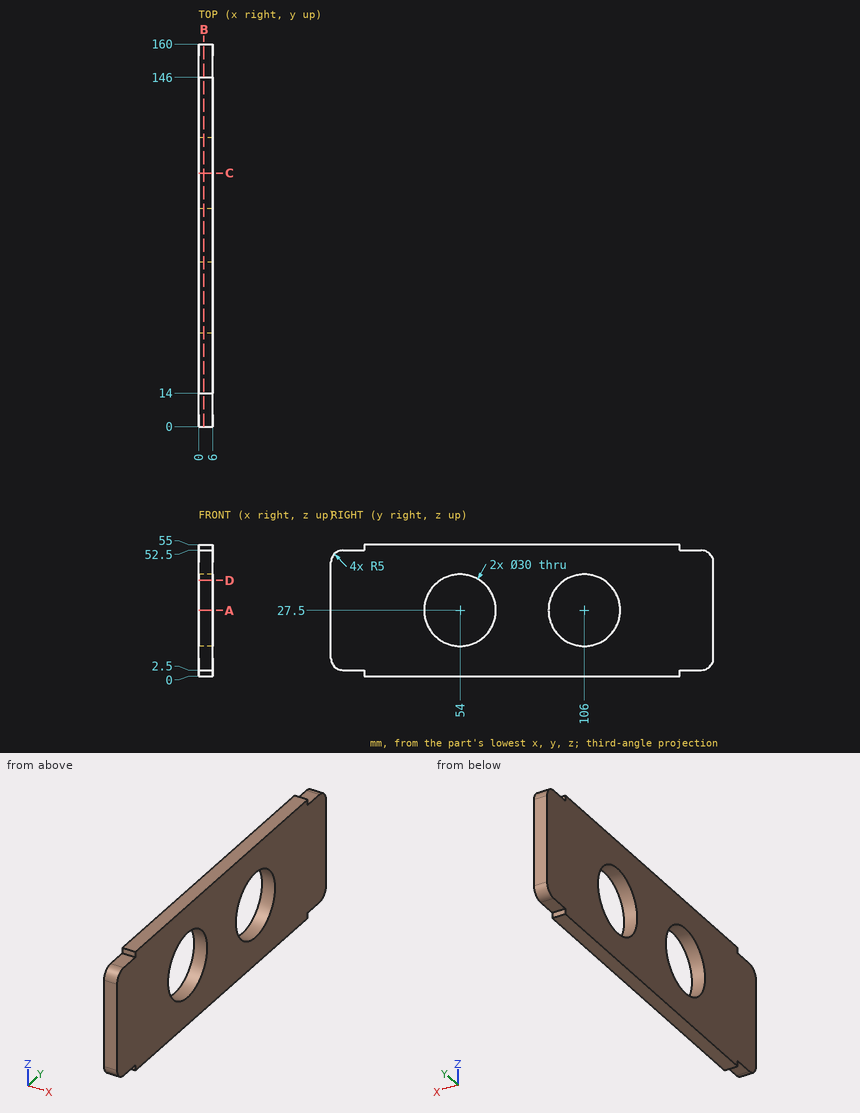
Part print with two shaded views. Sizes in mm from the minimum x, y, z corner. Coordinates: 2 decimals unless noted, no trailing zeros. Write each loop counter-clockwise with the first axis right and the second up, starting at its lowest first coordinate (ties: lowest second). Pieces come first, ordered by that corner, then holes. Notation, with made-up numbers: (55, 79.25) -> (81, 79.25) arc R24 cw to (81, 93.25) -> close; hole circle Ø9 at (84, -4). An arc over 180 degrees is marked (long way). Return JSON: item names as keys, results as strings. Group by question number.
Q1. Cut at B-B, the plane x = 2.2. Give the cut face in (y, z), then the cut area to 3 significant figures.
Q2. Cut at A-A, the plane z = 27.5. Give the cut face in (x, y).
Q3. Cut at D-D, the plane z = 40. Give the cut face in (x, y).
Q4. Drill centre lines: line 1 (Y direction, x = 2.3, z = 28); line 2 (Y direction, x = 4.25, z = 22.5); line 3 (Z direction, x = 3.95, y = 105). Where is each one in solid material? Low to high.
Q5. Cut at C-C, the plane y = 106. Give the cut face in (x, z), then the cut area to 3 significant figures.
Q6. Flat gauge pins, fed straight in: pin 1 (3 mm diameter, centred on x = 2.5, y = 150.5, fed in from -Z); pin 2 (18 mm diameter, centred on y = 106, z = 27.5, fed in from +X); pin 3 (0.8 mm diameter, centred on x = 3, z = 54, fed in from +Y); pin 4 (1.2 mm diameter, centred on x = 3, z = 54, fed in from -Y). Where does each tip first touch, or does it go through?
Returned:
{
 "1": {"outline": "(0, 7.5) arc R5 ccw to (5, 2.5) -> (14, 2.5) -> (14, 0) -> (146, 0) -> (146, 2.5) -> (155, 2.5) arc R5 ccw to (160, 7.5) -> (160, 47.5) arc R5 ccw to (155, 52.5) -> (146, 52.5) -> (146, 55) -> (14, 55) -> (14, 52.5) -> (5, 52.5) arc R5 ccw to (0, 47.5) -> close; hole circle Ø30 at (54, 27.5); hole circle Ø30 at (106, 27.5)", "area": "7,220 mm2"},
 "2": {"outline": "(0, 0) -> (6, 0) -> (6, 39) -> (0, 39) -> close; (0, 69) -> (6, 69) -> (6, 91) -> (0, 91) -> close; (0, 121) -> (6, 121) -> (6, 160) -> (0, 160) -> close"},
 "3": {"outline": "(0, 0) -> (6, 0) -> (6, 45.71) -> (0, 45.71) -> close; (0, 62.29) -> (6, 62.29) -> (6, 97.71) -> (0, 97.71) -> close; (0, 114.29) -> (6, 114.29) -> (6, 160) -> (0, 160) -> close"},
 "4": {"line 1": "y = 0 to 39.01, 68.99 to 91.01, 120.99 to 160", "line 2": "y = 0 to 39.86, 68.14 to 91.86, 120.14 to 160", "line 3": "z = 0 to 12.53, 42.47 to 55"},
 "5": {"outline": "(0, 0) -> (6, 0) -> (6, 12.5) -> (0, 12.5) -> close; (0, 42.5) -> (6, 42.5) -> (6, 55) -> (0, 55) -> close", "area": "150 mm2"},
 "6": {"pin 1": "stops at z = 2.5", "pin 2": "passes through", "pin 3": "stops at y = 146", "pin 4": "stops at y = 14"}
}
